CAD build for the part. Positions are in the model's coordinates, mm. Face numbers are marked on the shaded views. A direction names the side the tool comes from. Coordinates: 2 decimals unless noted, no trailing zeros. Write each loop counter-clockwise with the first axis right and the second up, starting at its lowest first coordinate (ties: lowest second). Pieces come first, ordered by that corner, then holes. Notation, with made-up numbers: (21, 9.25) -> (52, 9.25) arc R19 ccw to (52, 31.25) -> close; hole circle Ø4 at (-17.5, 41.5). An arc over 180 degrees is marked (long way). Answer as CSV lines item,"result". Start each with the question number.
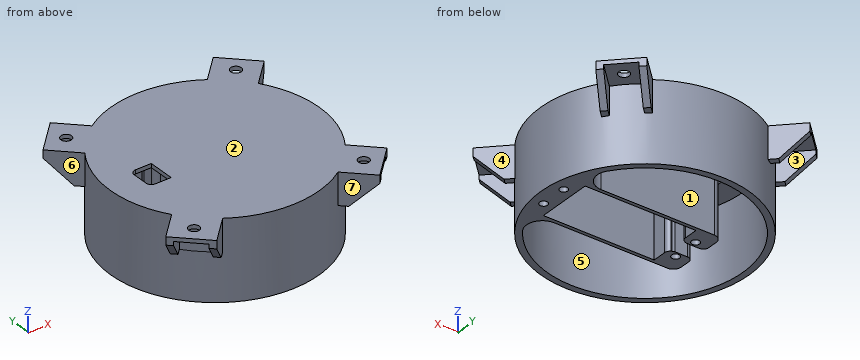
```python
from build123d import *

# Parameters (mm, degrees)
SKETCH1_R           = 39.5
BOSS_EXTRUDE1_DEPTH = 30.15
SKETCH3_W           = 42
SKETCH3_H           = 21
CUT_EXTRUDE1_DEPTH  = 28.65
CUT_EXTRUDE2_DEPTH  = 28.65
SKETCH5_R           = 1.5
CUT_EXTRUDE3_DEPTH  = 28.65
SKETCH8_W           = 8
SKETCH8_H           = 10
CUT_EXTRUDE5_DEPTH  = 76.391291937
FILLET1_R           = 3
FILLET3_R           = 6
FILLET2_R           = 2
SKETCH12_R          = 2
BOSS_EXTRUDE3_DEPTH = 12
CUT_EXTRUDE6_REACH  = 78.373
CUT_EXTRUDE7_DEPTH  = 10.5
CIRPATTERN19_COUNT  = 4


with BuildPart() as part:
    # Sketch1 → Boss-Extrude1 (new body)
    with BuildSketch(Plane.XY):
        with Locations(Location((-9.62, 10, 0), (0, 0, 180))):
            Circle(SKETCH1_R)
    extrude(amount=BOSS_EXTRUDE1_DEPTH)

    # Sketch3 → Cut-Extrude1 (cut)
    with BuildSketch(Plane(origin=(0, 0, 0), x_dir=(-1, 0, 0), z_dir=(0, 0, -1))):
        with Locations((0, 10)):
            Rectangle(SKETCH3_W, SKETCH3_H)
    extrude(amount=-CUT_EXTRUDE1_DEPTH, mode=Mode.SUBTRACT)

    # Sketch4 → Cut-Extrude2 (cut)
    with BuildSketch(Plane(origin=(0, 0, 0), x_dir=(-1, 0, 0), z_dir=(0, 0, -1))):
        with BuildLine():
            Line((30, -1.8), (-25.55342747, -1.8))
            ThreePointArc((-25.55342747, -1.8), (46.72, 10), (-25.55342747, 21.8))
            Line((-25.55342747, 21.8), (30, 21.8))
            Line((30, 21.8), (30, -1.8))
        make_face()
    extrude(amount=-CUT_EXTRUDE2_DEPTH, mode=Mode.SUBTRACT)

    # Sketch5 → Cut-Extrude3 (cut)
    with BuildSketch(Plane(origin=(0, 0, 0), x_dir=(-1, 0, 0), z_dir=(0, 0, -1))):
        with Locations((25, 4.96)):
            Circle(SKETCH5_R)
        with Locations((25, 15.04)):
            Circle(SKETCH5_R)
        with Locations((-25, 4.96)):
            Circle(SKETCH5_R)
        with Locations((-25, 15.04)):
            Circle(SKETCH5_R)
        Polygon((30, 7), (22.813409321, 7), (21, 6), (21, 7), (21, 13), (21, 14), (22.813409321, 13), (30, 13), align=None)
    extrude(amount=-CUT_EXTRUDE3_DEPTH, mode=Mode.SUBTRACT)

    # Sketch8 → Cut-Extrude5 (cut, through all)
    with BuildSketch(Plane(origin=(0, 0, 28.65), x_dir=(-1, 0, 0), z_dir=(0, 0, -1))):
        with Locations((34, 10)):
            Rectangle(SKETCH8_W, SKETCH8_H)
    extrude(amount=-CUT_EXTRUDE5_DEPTH, mode=Mode.SUBTRACT)

    # Fillet1
    fillet1_edges = [part.edges().sort_by_distance(p)[0] for p in [
        (-30, -1.8, 14.325),
        (-30, 21.8, 14.325),
    ]]
    fillet(fillet1_edges, radius=FILLET1_R)

    # Fillet3
    fillet3_edges = [part.edges().sort_by_distance(p)[0] for p in [
        (25.55342747, 21.8, 14.325),
        (25.55342747, -1.8, 14.325),
    ]]
    fillet(fillet3_edges, radius=FILLET3_R)

    # Fillet2
    fillet2_edges = [part.edges().sort_by_distance(p)[0] for p in [
        (-30, 13, 14.325),
        (-30, 7, 14.325),
        (-22.813409321, 7, 14.325),
        (-21, 6, 14.325),
        (-21, 14, 14.325),
        (-22.813409321, 13, 14.325),
        (-38, 15, 29.4),
        (-38, 5, 29.4),
    ]]
    fillet(fillet2_edges, radius=FILLET2_R)


with BuildPart() as body_2:
    # Sketch12 → Boss-Extrude3 (new body)
    with BuildSketch(Plane.XY.offset(30.15)):
        with BuildLine():
            Line((22.915425491, -11.504559705), (32.311432124, -20.900566338))
            Line((32.311432124, -20.900566338), (21.280566338, -31.931432124))
            Line((21.280566338, -31.931432124), (11.884559705, -22.535425491))
            ThreePointArc((11.884559705, -22.535425491), (17.957164466, -17.577164466), (22.915425491, -11.504559705))
        make_face()
        with Locations((22.553358544, -22.173358544)):
            Circle(SKETCH12_R, mode=Mode.SUBTRACT)
    extrude(amount=-BOSS_EXTRUDE3_DEPTH)

    # Cut-Extrude6: up to this face of the body (flat: up to its plane)
    cut_extrude6_end = Plane(body_2.part.faces().sort_by_distance((27.613428808, -16.202563021, 24.15))[0])
    # Sketch13 → Cut-Extrude6 (cut, up to the picked face)
    with BuildSketch(Plane(origin=(-5.325432893, -5.325432893, 0), x_dir=(0, 0, 1), z_dir=(-0.7071067811865415, -0.7071067811865537, 0)), mode=Mode.PRIVATE) as cut_extrude6_sk1:
        Polygon((18.15, -37.626564953), (27.15, -37.626564953), (18.15, -28.126564953), align=None)
    cut_extrude6_tool1 = split(extrude(cut_extrude6_sk1.sketch, amount=-CUT_EXTRUDE6_REACH, mode=Mode.PRIVATE), bisect_by=cut_extrude6_end, keep=Keep.BOTH, mode=Mode.PRIVATE)
    add(cut_extrude6_tool1.solids().sort_by(Axis((19.041395, -29.692261, 21.15), (0.7071067811865415, 0.7071067811865537, 0)))[0], mode=Mode.SUBTRACT)

    # Sketch14 → Cut-Extrude7 (cut)
    with BuildSketch(Plane(origin=(0, 0, 18.15), x_dir=(-1, 0, 0), z_dir=(0, 0, -1))):
        with BuildLine():
            Line((-14.230107258, -21.486860494), (-22.977622613, -30.23437585))
            Line((-22.977622613, -30.23437585), (-30.61437585, -22.597622613))
            Line((-30.61437585, -22.597622613), (-21.866860494, -13.850107258))
            ThreePointArc((-21.866860494, -13.850107258), (-18.310717857, -17.930717857), (-14.230107258, -21.486860494))
        make_face()
    extrude(amount=-CUT_EXTRUDE7_DEPTH, mode=Mode.SUBTRACT)


with BuildPart() as cirpattern19_1:
    # CirPattern19: pattern copy
    add(body_2.part.rotate(Axis((-9.62, 10, 0), (0, 0, 1)), 1 * 360 / CIRPATTERN19_COUNT))


with BuildPart() as cirpattern19_2:
    # CirPattern19: pattern copy
    add(body_2.part.rotate(Axis((-9.62, 10, 0), (0, 0, 1)), 2 * 360 / CIRPATTERN19_COUNT))


with BuildPart() as cirpattern19_3:
    # CirPattern19: pattern copy
    add(body_2.part.rotate(Axis((-9.62, 10, 0), (0, 0, 1)), 3 * 360 / CIRPATTERN19_COUNT))


with BuildPart() as part_1:
    add(part.part)

    # Combine1: union body 2, CirPattern19_3, CirPattern19_2, CirPattern19_1
    add(body_2.part)
    add(cirpattern19_3.part)
    add(cirpattern19_2.part)
    add(cirpattern19_1.part)


solid = part_1.part
```
1. Mould opens along X. For the marked faces 1, 2, 3 and 4 say: pulls with the +X half, pulls with the -X half, needs draft (parallel to the pull), parting line crosses it, or undercut.
2. Cut at B-B (z = 6.5). Count the separate pieces of the cut face and the enclosed holes in it, then the cut area to 3 significant figures.
3. Wall check: line 1 (Y direction, x = -9, z = 15); line 2 (X direction, y = 9, z = 5.5); line 3 (Y direction, x = 4, z = 6). Give the ranges that are in metal, low to high.
4. Cut at C-C (x = -9.62). Give the cut face in (y, z), then the cut area to 3 significant figures.
5. Cut at D-D (y = 25). Give the cut face in (x, z).
6. Flat gauge pins, fed straight in: P1, Ø12, axis at y = 27.5, z = 13.5, coming from the +X side; P2, Ø5, axis at x = -45, y = 43.5, coming from the -Z side; P3, Ø10, axis at x = -4.5, z = 23.5, coming from the -Y side; P4, Ø3, axis at x = 22.55, y = -22.17, coming from the +Z side. Where does each tip first touch, or does it go through?
7. Cut at A-A (y = 10). Give the cut face in (x, z), then the cut area to 3 significant figures.
8. Tool access for the marked faces 5, 6 and 7: list every direction of +Z, -Z, +X, -X, +Y, -Y with a clear straight run to the whole face (end or side of a thin tool).
Geometry check:
1,face 1,"undercut"
1,face 2,"needs draft"
1,face 3,"undercut"
1,face 4,"pulls with the +X half"
2,separate pieces,"1"
2,enclosed holes,"5"
2,area,"995 mm²"
3,line 1,"-29.5 to -27.09, -1.8 to -0.5, 20.5 to 21.8, 47.09 to 49.5"
3,line 2,"-49.11 to -46.71, 21 to 29.87"
3,line 3,"-27.08 to -24.51, -1.8 to -0.5, 20.5 to 21.8, 44.51 to 47.08"
4,outline,"(-29.5, 0) -> (-27.1, 0) -> (-27.1, 28.65) -> (-1.8, 28.65) -> (-1.8, 0) -> (-0.5, 0) -> (-0.5, 28.65) -> (20.5, 28.65) -> (20.5, 0) -> (21.8, 0) -> (21.8, 28.65) -> (47.1, 28.65) -> (47.1, 0) -> (49.5, 0) -> (49.5, 30.15) -> (-29.5, 30.15) -> close"
4,area,"331 mm²"
5,outline,"(-46.16, 0) -> (-43.55, 0) -> (-43.55, 28.65) -> (21.19, 28.65) -> (21.19, 0) -> (26.92, 0) -> (26.92, 30.15) -> (-46.16, 30.15) -> close"
6,P1,"x = 28.17"
6,P2,"z = 28.65"
6,P3,"y = -29.5"
6,P4,"through"
7,outline,"(-49.12, 0) -> (-46.72, 0) -> (-46.72, 28.65) -> (-38, 28.65) -> (-38, 30.15) -> (-49.12, 30.15) -> close; (-30, 28.65) -> (21, 28.65) -> (21, 0) -> (29.88, 0) -> (29.88, 30.15) -> (-30, 30.15) -> close"
7,area,"430 mm²"
8,face 5,"-Z"
8,face 6,"+Z, -Z, -X"
8,face 7,"+Z, -Z, -Y"
